Check sheet for the drawn part. Datum: minimum x, y, z corner. Units: mm. Give positions to 0.01 mm unless a question says otherwise; leave off trailing zeros. Loops run counter-clockwise (first coordinate to the right, second up) from the corner with the lowest first, then second, coordinate; pieces in that order, holes last. Notation, with made-up numbers: (-26, 62.25) - (25, 62.25) arc R21 cw to (25, 88.25) - close; hole circle Ø8 at (46.5, 32). An arc over 180 degrees is marked (long way). Use one line per item in the form item = value.
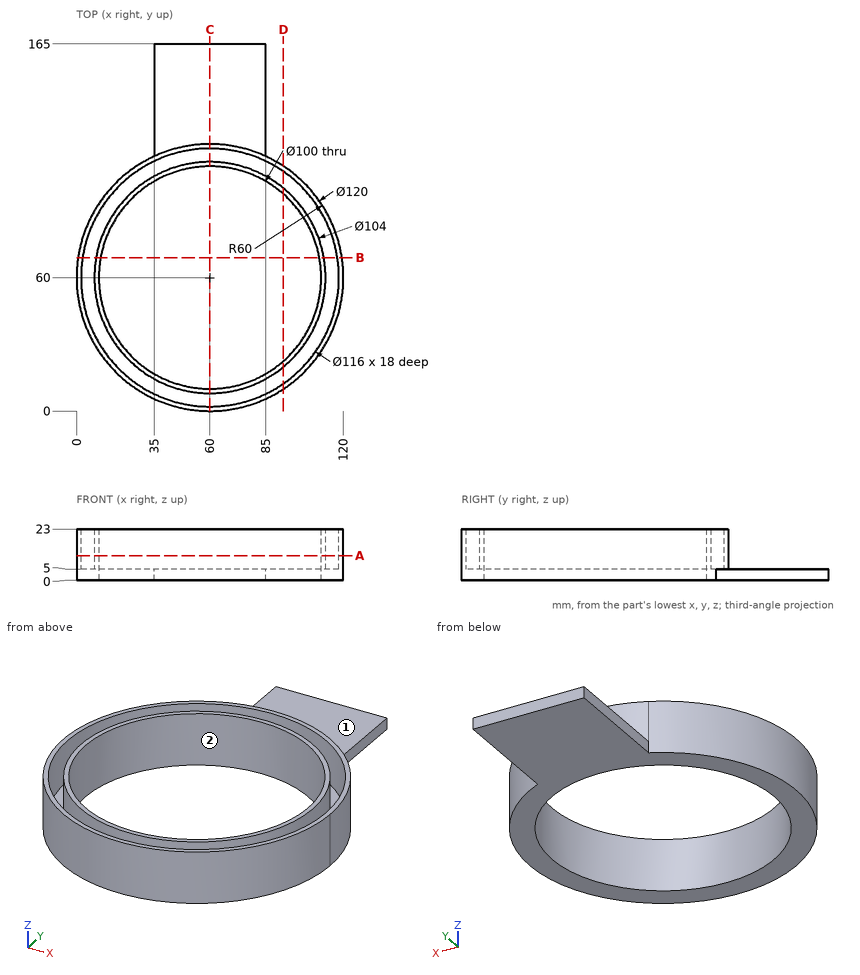
1. Draft check along X on the marked faces 1 and 2. Enter one of: released by +X, released by -X, zero draft, split by the parting line, or undercut.
Result set:
face_1 = zero draft
face_2 = undercut
2. Section check D-D, the plane x = 93. Record the cut outline in (y, z).
Result set:
outline = (9.89, 0) - (22.44, 0) - (22.44, 23) - (19.81, 23) - (19.81, 5) - (12.3, 5) - (12.3, 23) - (9.89, 23) - close; (97.56, 0) - (110.11, 0) - (110.11, 23) - (107.7, 23) - (107.7, 5) - (100.19, 5) - (100.19, 23) - (97.56, 23) - close
3. Section check A-A, the plane z = 11. Record the cut outline in (x, y), then the cut area to 3 significant figures.
Result set:
outline = circle Ø104 at (60, 60); (35, 114.54) arc R60 ccw (long way) to (120, 60) arc R60 ccw to (85, 114.54) arc R60 ccw to start; hole circle Ø116 at (60, 60); hole circle Ø100 at (60, 60)
area = 1,380 mm²
4. Section check C-C, the plane x = 60. Record the cut outline in (y, z), then the cut area to 3 significant figures.
Result set:
outline = (0, 0) - (10, 0) - (10, 23) - (8, 23) - (8, 5) - (2, 5) - (2, 23) - (0, 23) - close; (110, 0) - (165, 0) - (165, 5) - (120, 5) - (120, 23) - (118, 23) - (118, 5) - (112, 5) - (112, 23) - (110, 23) - close
area = 469 mm²
5. Depth check by flat-ended pin: pin 1 Ø4 at (y, z) = (134, 2.5) entering from +X; pin 2 Ø1.5 at (y, z) = (145.5, 3) entering from -X; pin 3 Ø3 at (y, z) = (54, 7.5) entering from +X; pin 4 Ø1 at (x, y) = (14.5, 77.5) entering from -Z. Enter the tip coordinate at first touch or a pass-through.
Result set:
pin_1 = 85
pin_2 = 35
pin_3 = 119.83
pin_4 = through
6. Section check B-B, the plane y = 69. Record the cut outline in (x, z).
Result set:
outline = (0.68, 0) - (10.82, 0) - (10.82, 23) - (8.78, 23) - (8.78, 5) - (2.7, 5) - (2.7, 23) - (0.68, 23) - close; (109.18, 0) - (119.32, 0) - (119.32, 23) - (117.3, 23) - (117.3, 5) - (111.22, 5) - (111.22, 23) - (109.18, 23) - close
7. Scan lines: probe 1 along Y at (x, z) = (60, 18.5); probe 2 along Y at (x, z) = (68.5, 10.75). Record each from-to range of solid material in increasing order.
Result set:
probe_1 = 0 to 2, 8 to 10, 110 to 112, 118 to 120
probe_2 = 0.61 to 2.63, 8.7 to 10.73, 109.27 to 111.3, 117.37 to 119.39
